Read the model definition and answer for the solid it produces. Units are mm, in the model's axes. Face numbers are marked on the shaded views. Round coordinates to 2 decimals unless told otherwise and drop trailing zeros. Loops run counter-clockwise (first coordinate to the right, second up) from the corner with the lowest first, then second, coordinate; pieces in that order, holes last. Notation, with made-up numbers: M 33.5,-2.75 L 53.5,-2.75 A10 cw 53.5,11.25 Z; hole C -11.75,42 d11. An arc over 180 degrees is marked long. Answer as CSV lines item,"result".
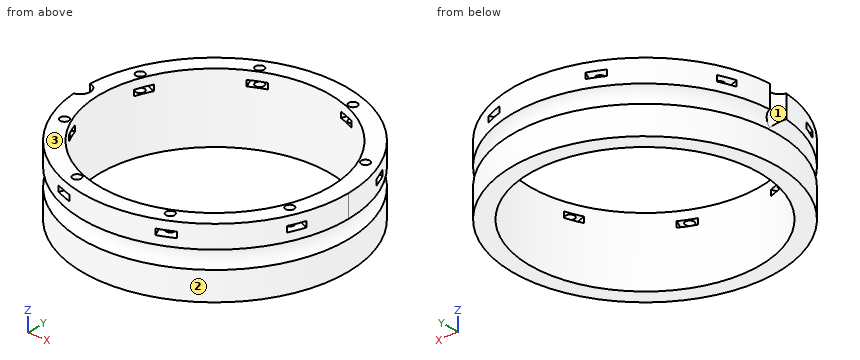
```python
from build123d import *

# Parameters (mm, degrees)
BOX445_W                     = 6
BOX445_H                     = 8
BOX445_DEPTH                 = 2
BOX445_PLACEMENT_ANGLE       = 45
BOX443_W                     = 6
BOX443_H                     = 8
BOX443_DEPTH                 = 2
BOX442_W                     = 6
BOX442_H                     = 8
BOX442_DEPTH                 = 2
BOX447_W                     = 6
BOX447_H                     = 8
BOX447_DEPTH                 = 2
BOX447_PLACEMENT_ANGLE       = 135
BOX446_W                     = 6
BOX446_H                     = 8
BOX446_DEPTH                 = 2
BOX441_W                     = 6
BOX441_H                     = 8
BOX441_DEPTH                 = 2
BOX441_PLACEMENT_ANGLE       = 225
BOX444_W                     = 6
BOX444_H                     = 8
BOX444_DEPTH                 = 2
BOX437_W                     = 6
BOX437_H                     = 8
BOX437_DEPTH                 = 2
BOX437_PLACEMENT_ANGLE       = 45
COMPOUND869_PLACEMENT_ANGLE  = 22.5
CYLINDER1133_R               = 1.5
CYLINDER1133_DEPTH           = 32
CYLINDER1133_PLACEMENT_ANGLE = 45
CYLINDER1132_R               = 1.5
CYLINDER1132_DEPTH           = 32
CYLINDER1131_R               = 1.5
CYLINDER1131_DEPTH           = 32
CYLINDER1131_PLACEMENT_ANGLE = 135
CYLINDER1123_R               = 1.5
CYLINDER1123_DEPTH           = 32
CYLINDER1129_R               = 1.5
CYLINDER1129_DEPTH           = 32
CYLINDER1129_PLACEMENT_ANGLE = 225
CYLINDER1130_R               = 1.5
CYLINDER1130_DEPTH           = 32
CYLINDER1118_R               = 1.5
CYLINDER1118_DEPTH           = 32
CYLINDER1118_PLACEMENT_ANGLE = 45
CYLINDER1121_R               = 1.5
CYLINDER1121_DEPTH           = 32
COMPOUND871_PLACEMENT_ANGLE  = 22.5
CYLINDER1114_R               = 3.5
CYLINDER1114_DEPTH           = 20
TORUS009_R                   = 3.1
TUBE100_R                    = 46
TUBE100_R_2                  = 40
TUBE100_DEPTH                = 24


with BuildPart() as krychle445:
    # Box445 → Box445 (new body)
    with BuildSketch(Plane.XY):
        with Locations((3, 4)):
            Rectangle(BOX445_W, BOX445_H)
    extrude(amount=BOX445_DEPTH)


with BuildPart() as krychle445_1:
    # Box445 placement: moved
    add(krychle445.part.moved(Location((30.405592, -34.648232, 33))).rotate(Axis((30.405592, -34.648232, 33), (0, 0, 1)), BOX445_PLACEMENT_ANGLE))


with BuildPart() as krychle443:
    # Box443 → Box443 (new body)
    with BuildSketch(Plane(origin=(46, -3, 33), x_dir=(0, 1, 0), z_dir=(0, 0, 1))):
        with Locations((3, 4)):
            Rectangle(BOX443_W, BOX443_H)
    extrude(amount=BOX443_DEPTH)


with BuildPart() as krychle442:
    # Box442 → Box442 (new body)
    with BuildSketch(Plane(origin=(-3, -46, 33), x_dir=(1, 0, 0), z_dir=(0, 0, 1))):
        with Locations((3, 4)):
            Rectangle(BOX442_W, BOX442_H)
    extrude(amount=BOX442_DEPTH)


with BuildPart() as krychle447:
    # Box447 → Box447 (new body)
    with BuildSketch(Plane.XY):
        with Locations((3, 4)):
            Rectangle(BOX447_W, BOX447_H)
    extrude(amount=BOX447_DEPTH)


with BuildPart() as krychle447_1:
    # Box447 placement: moved
    add(krychle447.part.moved(Location((34.648232, 30.405592, 33))).rotate(Axis((34.648232, 30.405592, 33), (0, 0, 1)), BOX447_PLACEMENT_ANGLE))


with BuildPart() as krychle446:
    # Box446 → Box446 (new body)
    with BuildSketch(Plane(origin=(3, 46, 33), x_dir=(-1, 0, 0), z_dir=(0, 0, 1))):
        with Locations((3, 4)):
            Rectangle(BOX446_W, BOX446_H)
    extrude(amount=BOX446_DEPTH)


with BuildPart() as krychle441:
    # Box441 → Box441 (new body)
    with BuildSketch(Plane.XY):
        with Locations((3, 4)):
            Rectangle(BOX441_W, BOX441_H)
    extrude(amount=BOX441_DEPTH)


with BuildPart() as krychle441_1:
    # Box441 placement: moved
    add(krychle441.part.moved(Location((-30.405592, 34.648232, 33))).rotate(Axis((-30.405592, 34.648232, 33), (0, 0, 1)), BOX441_PLACEMENT_ANGLE))


with BuildPart() as krychle444:
    # Box444 → Box444 (new body)
    with BuildSketch(Plane(origin=(-46, 3, 33), x_dir=(0, -1, 0), z_dir=(0, 0, 1))):
        with Locations((3, 4)):
            Rectangle(BOX444_W, BOX444_H)
    extrude(amount=BOX444_DEPTH)


with BuildPart() as compound869:
    # Box437 → Box437 (new body)
    with BuildSketch(Plane.XY):
        with Locations((3, 4)):
            Rectangle(BOX437_W, BOX437_H)
    extrude(amount=BOX437_DEPTH)


with BuildPart() as compound869_1:
    # Box437 placement: moved
    add(compound869.part.moved(Location((-34.648232, -30.405592, 33))).rotate(Axis((-34.648232, -30.405592, 33), (0, 0, -1)), BOX437_PLACEMENT_ANGLE))

    # Compound869: union Krychle445, Krychle443, Krychle442, Krychle447, Krychle446, Krychle441, Krychle444
    add(krychle445_1.part)
    add(krychle443.part)
    add(krychle442.part)
    add(krychle447_1.part)
    add(krychle446.part)
    add(krychle441_1.part)
    add(krychle444.part)


with BuildPart() as compound869_2:
    # Compound869 placement: moved
    add(compound869_1.part.moved(Location((0, 0, 7))).rotate(Axis((0, 0, 7), (0, 0, 1)), COMPOUND869_PLACEMENT_ANGLE))


with BuildPart() as obj1:
    # Cylinder1133 → Cylinder1133 (new body)
    with BuildSketch(Plane.XY):
        Circle(CYLINDER1133_R)
    extrude(amount=CYLINDER1133_DEPTH)


with BuildPart() as obj1_1:
    # Cylinder1133 placement: moved
    add(obj1.part.moved(Location((29.698485, -29.698485, 33.5))).rotate(Axis((29.698485, -29.698485, 33.5), (0, 0, 1)), CYLINDER1133_PLACEMENT_ANGLE))


with BuildPart() as obj2:
    # Cylinder1132 → Cylinder1132 (new body)
    with BuildSketch(Plane(origin=(42, 0, 33.5), x_dir=(0, 1, 0), z_dir=(0, 0, 1))):
        Circle(CYLINDER1132_R)
    extrude(amount=CYLINDER1132_DEPTH)


with BuildPart() as obj3:
    # Cylinder1131 → Cylinder1131 (new body)
    with BuildSketch(Plane.XY):
        Circle(CYLINDER1131_R)
    extrude(amount=CYLINDER1131_DEPTH)


with BuildPart() as obj3_1:
    # Cylinder1131 placement: moved
    add(obj3.part.moved(Location((29.698485, 29.698485, 33.5))).rotate(Axis((29.698485, 29.698485, 33.5), (0, 0, 1)), CYLINDER1131_PLACEMENT_ANGLE))


with BuildPart() as obj4:
    # Cylinder1123 → Cylinder1123 (new body)
    with BuildSketch(Plane(origin=(0, 42, 33.5), x_dir=(-1, 0, 0), z_dir=(0, 0, 1))):
        Circle(CYLINDER1123_R)
    extrude(amount=CYLINDER1123_DEPTH)


with BuildPart() as obj5:
    # Cylinder1129 → Cylinder1129 (new body)
    with BuildSketch(Plane.XY):
        Circle(CYLINDER1129_R)
    extrude(amount=CYLINDER1129_DEPTH)


with BuildPart() as obj5_1:
    # Cylinder1129 placement: moved
    add(obj5.part.moved(Location((-29.698485, 29.698485, 33.5))).rotate(Axis((-29.698485, 29.698485, 33.5), (0, 0, 1)), CYLINDER1129_PLACEMENT_ANGLE))


with BuildPart() as obj6:
    # Cylinder1130 → Cylinder1130 (new body)
    with BuildSketch(Plane(origin=(-42, 0, 33.5), x_dir=(0, -1, 0), z_dir=(0, 0, 1))):
        Circle(CYLINDER1130_R)
    extrude(amount=CYLINDER1130_DEPTH)


with BuildPart() as obj7:
    # Cylinder1118 → Cylinder1118 (new body)
    with BuildSketch(Plane.XY):
        Circle(CYLINDER1118_R)
    extrude(amount=CYLINDER1118_DEPTH)


with BuildPart() as obj7_1:
    # Cylinder1118 placement: moved
    add(obj7.part.moved(Location((-29.698485, -29.698485, 33.5))).rotate(Axis((-29.698485, -29.698485, 33.5), (0, 0, -1)), CYLINDER1118_PLACEMENT_ANGLE))


with BuildPart() as compound871:
    # Cylinder1121 → Cylinder1121 (new body)
    with BuildSketch(Plane(origin=(0, -42, 33.5), x_dir=(1, 0, 0), z_dir=(0, 0, 1))):
        Circle(CYLINDER1121_R)
    extrude(amount=CYLINDER1121_DEPTH)

    # Compound871: union obj1, obj2, obj3, obj4, obj5, obj6, obj7
    add(obj1_1.part)
    add(obj2.part)
    add(obj3_1.part)
    add(obj4.part)
    add(obj5_1.part)
    add(obj6.part)
    add(obj7_1.part)


with BuildPart() as compound871_1:
    # Compound871 placement: moved
    add(compound871.part.moved(Location((0, 0, 4))).rotate(Axis((0, 0, 4), (0, 0, 1)), COMPOUND871_PLACEMENT_ANGLE))


with BuildPart() as obj8:
    # Cylinder1114 → Cylinder1114 (new body)
    with BuildSketch(Plane(origin=(-46.4, 0, 34), x_dir=(1, 0, 0), z_dir=(0, 0, 1))):
        Circle(CYLINDER1114_R)
    extrude(amount=CYLINDER1114_DEPTH)


with BuildPart() as obj9:
    # Torus009 → Torus009 (revolve)
    with BuildSketch(Plane(origin=(0, 0, 34), x_dir=(1, 0, 0), z_dir=(0, -1, 0))):
        with Locations((46, 0)):
            Circle(TORUS009_R)
    revolve(axis=Axis((0, 0, 34), (0, 0, 1)))


with BuildPart() as cut421:
    # Tube100 → Tube100 (new body)
    with BuildSketch(Plane.XY.offset(21)):
        Circle(TUBE100_R)
        Circle(TUBE100_R_2, mode=Mode.SUBTRACT)
    extrude(amount=TUBE100_DEPTH)

    # Cut419: cut obj9
    add(obj9.part, mode=Mode.SUBTRACT)

    # Cut426: cut obj8
    add(obj8.part, mode=Mode.SUBTRACT)

    # Cut420: cut Compound871
    add(compound871_1.part, mode=Mode.SUBTRACT)

    # Cut421: cut Compound869
    add(compound869_2.part, mode=Mode.SUBTRACT)


solid = cut421.part
```
1) Determine the mould class of the marked faces 1, 2 and 3 for opening direction Y: released by +Y, released by -Y, zero draft, split by the parting line, or undercut.
Evaluation:
face 1,"undercut"
face 2,"split by the parting line"
face 3,"zero draft"
2) Each of these flat-tipped pins is pushed along its axis until it touches: P1, Ø3, axis at x = 2.5, z = 27, coming from the -Y side; P2, Ø2.5, axis at x = 38.8, y = -16.07, coming from the +Z side; P3, Ø2, axis at x = 11.5, z = 31, coming from the +Y side. Where does it stop, or does it pass through?
Evaluation:
P1,"stops at y = -45.99"
P2,"stops at z = 37.5"
P3,"stops at y = 44.78"
3) Straight lines are drawn through the part: line 1 (Z direction, x = -36, y = -18); line 2 (X direction, y = -25, z = 35.5); line 3 (X direction, y = 9, z = 41.75). For each, find the intervals that lie inside material, in ascending order.
Evaluation:
line 1,"z = 21 to 40, 42 to 45"
line 2,"x = -35.34 to -31.22, 31.22 to 35.34"
line 3,"x = -45.11 to -38.97, 38.97 to 45.11"
4) Find section B-B, the plane z = 24.5. Give the vertices of the cut face in (x, y).
Evaluation:
outline,"C 0,0 d92; hole C 0,0 d80"
5) Find section A-A, the plane x = 0. Give the vertices of the cut face in (y, z), then the cut area to 3 significant figures.
Evaluation:
outline,"M -46,21 L -40,21 L -40,45 L -46,45 L -46,37.1 A3.1 cw -46,30.9 Z; M 40,21 L 46,21 L 46,30.9 A3.1 cw 46,37.1 L 46,45 L 40,45 Z"
area,"258 mm^2"
